```python
from build123d import *

# Parameters (mm, degrees)
FILLET1_R   = 0.8
HEX_2_DEPTH = 5.6


with BuildPart() as part:
    # BodySke → BaseBody (revolve)
    with BuildSketch(Plane.XY):
        Polygon((0, 0), (0, 4), (0.3, 4), (2.3, 2), (17.8, 2), (18.3, 1.5), (18.3, 0), align=None)
    revolve(axis=Axis((0, 0, 0), (1, 0, 0)))

    # Fillet1
    fillet1_edges = [part.edges().sort_by_distance(p)[0] for p in [
        (2.3, -2, 0),
    ]]
    fillet(fillet1_edges, radius=FILLET1_R)

    # Sketch3 → Hex 2 (cut)
    with BuildSketch(Plane.ZY):
        Polygon((-1.25, -0.721687836), (-1.25, 0.721687836), (0, 1.443375673), (1.25, 0.721687836), (1.25, -0.721687836), (0, -1.443375673), align=None)
    extrude(amount=-HEX_2_DEPTH, mode=Mode.SUBTRACT)


solid = part.part
```
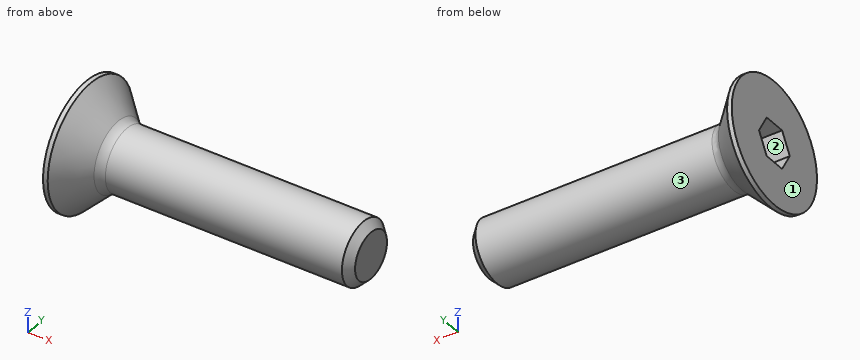
Geometry check sheet. Reference: the model listing, model coordinates, mm. Face numbers are marked on the shaded views. Coordinates: 2 decimals unless noted, no trailing zeros. Loops run counter-clockwise (first coordinate to the right, second up) from the corner with the lowest first, then second, coordinate; pieces in that order, holes last.
Item 1: Sectioned sample at B-B, the plane x = 9.75. Record the boundary of the cut face in (y, z), then the cut area to 3 significant figures.
Item 2: Release check for a two-part mould opening along Z. For the marked faces 1, 2 and 3 record: released by +Z, released by -Z, zero draft, split by the parting line, or undercut.
Item 3: Go/stop test with flat-tipped pins: pin 1 Ø1 at (x, y) = (9.5, 0.5) entering from +Z; pin 2 Ø3 at (y, z) = (0, 0) entering from -X; pin 3 Ø0.7 at (x, y) = (4, 0) entering from -Z; pin 4 Ø2 at (x, z) = (3, 2.5) entering from +Y. Record where each tip stops, or that it passes through.
Item 4: Thickness scan on line 1 (Y direction, x = 10.5, z = 0); line 2 (X direction, y = -0.5, z = -2.25). Record the ranges inside material, lowest first.
Item 5: Sectioned sample at A-A, the plane x = 3. Record the boundary of the cut face in (y, z).
Check result:
1. outline: circle Ø4 at (0, 0)
1. area: 12.6 mm2
2. face 1: zero draft
2. face 2: undercut
2. face 3: split by the parting line
3. pin 1: stops at z = 2
3. pin 2: stops at x = 0
3. pin 3: stops at z = -2
3. pin 4: stops at y = 1.32
4. line 1: y = -2 to 2
4. line 2: x = 0 to 2
5. outline: circle Ø4 at (0, 0); hole (-1.44, 0) - (-0.72, -1.25) - (0.72, -1.25) - (1.44, 0) - (0.72, 1.25) - (-0.72, 1.25) - close
